from build123d import *

# Parameters (mm, degrees)
SKETCH1_W           = 62.4
SKETCH1_H           = 72.4
SKETCH1_R           = 1.55
SKETCH1_W_2         = 14
BOSS_EXTRUDE1_DEPTH = 1.5
SKETCH3_W           = 14.75
SKETCH3_H           = 25
SKETCH3_W_2         = 12.75
SKETCH3_H_2         = 23
BOSS_EXTRUDE2_DEPTH = 3
SKETCH4_W           = 4
SKETCH4_H           = 4
BOSS_EXTRUDE3_DEPTH = 16.5
SKETCH5_R           = 0.875
CUT_EXTRUDE1_DEPTH  = 4
FILLET1_R           = 1
SKETCH6_R           = 1.55
CUT_EXTRUDE5_DEPTH  = 61.214034909
SKETCH7_W           = 5
SKETCH7_H           = 20
CUT_EXTRUDE3_DEPTH  = 61.214034909
SKETCH8_R           = 1.5
CUT_EXTRUDE4_DEPTH  = 61.64222951
SKETCH9_R           = 1.636711996
CUT_EXTRUDE6_DEPTH  = 61.214034909


with BuildPart() as part:
    # Sketch1 → Boss-Extrude1 (new body)
    # profile 1 of 2: a face of its own
    with BuildSketch(Plane(origin=(0, 0, 0), x_dir=(1, 0, 0), z_dir=(0, 1, 0))):
        Rectangle(SKETCH1_W, SKETCH1_H)
        with Locations(Location((-27.333, -32.333, 0), (0, 0, 270))):
            Circle(SKETCH1_R, mode=Mode.SUBTRACT)
        with Locations(Location((27.333, -32.333, 0), (0, 0, 270))):
            Circle(SKETCH1_R, mode=Mode.SUBTRACT)
        with Locations(Location((-27.333, 32.333, 0), (0, 0, 270))):
            Circle(SKETCH1_R, mode=Mode.SUBTRACT)
        with Locations(Location((27.333, 32.333, 0), (0, 0, 270))):
            Circle(SKETCH1_R, mode=Mode.SUBTRACT)
    # profile 2 of 2: a face of its own
    with BuildSketch(Plane(origin=(0, 0, 0), x_dir=(1, 0, 0), z_dir=(0, 1, 0))):
        with Locations((38.2, 0)):
            Rectangle(SKETCH1_W_2, SKETCH1_H)
    extrude(amount=BOSS_EXTRUDE1_DEPTH)

    # Sketch3 → Boss-Extrude2 (add)
    with BuildSketch(Plane(origin=(0, 1.5, 0), x_dir=(1, 0, 0), z_dir=(0, 1, 0))):
        with Locations((37.825, 0)):
            Rectangle(SKETCH3_W, SKETCH3_H)
        with Locations((37.825, 0)):
            Rectangle(SKETCH3_W_2, SKETCH3_H_2, mode=Mode.SUBTRACT)
    extrude(amount=BOSS_EXTRUDE2_DEPTH)

    # Sketch4 → Boss-Extrude3 (add)
    with BuildSketch(Plane(origin=(0, 1.5, 0), x_dir=(1, 0, 0), z_dir=(0, 1, 0))):
        with Locations((37.825, -14)):
            Rectangle(SKETCH4_W, SKETCH4_H)
        with Locations((37.825, 14.5)):
            Rectangle(SKETCH4_W, SKETCH4_H)
    extrude(amount=BOSS_EXTRUDE3_DEPTH)

    # Sketch5 → Cut-Extrude1 (cut)
    with BuildSketch(Plane(origin=(0, 18, 0), x_dir=(1, 0, 0), z_dir=(0, 1, 0))):
        with Locations(Location((37.825, -14, 0), (0, 0, 270))):
            Circle(SKETCH5_R)
        with Locations(Location((37.825, 14.5, 0), (0, 0, 270))):
            Circle(SKETCH5_R)
    extrude(amount=-CUT_EXTRUDE1_DEPTH, mode=Mode.SUBTRACT)

    # Fillet1
    fillet1_edges = [part.edges().sort_by_distance(p)[0] for p in [
        (42.5125, 1.5, -12.5),
        (30.45, 1.5, 0),
        (33.1375, 1.5, 12.5),
        (42.5125, 1.5, 12.5),
        (35.825, 1.5, 14.25),
        (39.825, 1.5, 14.25),
        (37.825, 1.5, 16),
        (33.1375, 1.5, -12.5),
        (35.825, 1.5, -14.5),
        (39.825, 1.5, -14.5),
        (37.825, 1.5, -16.5),
    ]]
    fillet(fillet1_edges, radius=FILLET1_R)

    # Sketch6 → Cut-Extrude5 (cut, through all)
    with BuildSketch(Plane(origin=(0, 1.5, 0), x_dir=(1, 0, 0), z_dir=(0, 1, 0))):
        with Locations(Location((7.473, -32.333, 0), (0, 0, 270))):
            Circle(SKETCH6_R)
        with Locations(Location((7.473, 32.333, 0), (0, 0, 270))):
            Circle(SKETCH6_R)
    extrude(amount=-CUT_EXTRUDE5_DEPTH, mode=Mode.SUBTRACT)

    # Sketch7 → Cut-Extrude3 (cut, through all)
    with BuildSketch(Plane(origin=(0, 1.5, 0), x_dir=(1, 0, 0), z_dir=(0, 1, 0))):
        with Locations((20, 0)):
            Rectangle(SKETCH7_W, SKETCH7_H)
    extrude(amount=-CUT_EXTRUDE3_DEPTH, mode=Mode.SUBTRACT)

    # Sketch8 → Cut-Extrude4 (cut, through all)
    with BuildSketch(Plane.XZ):
        with Locations(Location((-22.2, -6.73, 0), (0, 0, 270))):
            Circle(SKETCH8_R)
        with Locations(Location((-22.2, 6.73, 0), (0, 0, 270))):
            Circle(SKETCH8_R)
    extrude(amount=-CUT_EXTRUDE4_DEPTH, mode=Mode.SUBTRACT)

    # Sketch9 → Cut-Extrude6 (cut, through all)
    with BuildSketch(Plane(origin=(0, 1.5, 0), x_dir=(1, 0, 0), z_dir=(0, 1, 0))):
        with Locations(Location((-22.2, 6.73, 0), (0, 0, 270))):
            Circle(SKETCH9_R)
        with BuildLine():
            Line((-20.2, 24.2), (-20.2, 18.2))
            ThreePointArc((-20.2, 18.2), (-22.2, 16.2), (-24.2, 18.2))
            Line((-24.2, 18.2), (-24.2, 24.2))
            ThreePointArc((-24.2, 24.2), (-22.2, 26.2), (-20.2, 24.2))
        make_face()
        with BuildLine():
            Line((-20.2, -18.2), (-20.2, -24.2))
            ThreePointArc((-20.2, -24.2), (-22.2, -26.2), (-24.2, -24.2))
            Line((-24.2, -24.2), (-24.2, -18.2))
            ThreePointArc((-24.2, -18.2), (-22.2, -16.2), (-20.2, -18.2))
        make_face()
        with BuildLine():
            Line((10.8, 24.2), (10.8, 18.2))
            ThreePointArc((10.8, 18.2), (12.8, 16.2), (14.8, 18.2))
            Line((14.8, 18.2), (14.8, 24.2))
            ThreePointArc((14.8, 24.2), (12.8, 26.2), (10.8, 24.2))
        make_face()
        with BuildLine():
            Line((10.8, -18.2), (10.8, -24.2))
            ThreePointArc((10.8, -24.2), (12.8, -26.2), (14.8, -24.2))
            Line((14.8, -24.2), (14.8, -18.2))
            ThreePointArc((14.8, -18.2), (12.8, -16.2), (10.8, -18.2))
        make_face()
    extrude(amount=-CUT_EXTRUDE6_DEPTH, mode=Mode.SUBTRACT)


solid = part.part
Geometry check sheet. Reference: the model listing, model coordinates, mm. A direction names the side the tool comes from. Give positions to 0.01 mm unless a question says otherwise; leave off trailing zeros. Loops run counter-clockwise (first coordinate to the right, second up) from the corner with the lowest first, then second, coordinate; pieces in that order, holes last. Notation, with made-up numbers: M 10.5,36.5 L 57.5,36.5 A23 cw 57.5,54.5 Z; hole C 1,13.5 d3. An arc over 180 degrees is marked long. Answer as a JSON object with one key per item and string values. Group by question number.
Item 1: Sectioned sample at A-A on y = 12.25. Record the boundary of the cut face in (x, z) (3 decimals), plus the area to 3 significant figures.
Item 2: Gauge pin test, flat ends, axial feed: pin 1 (2 mm diameter, centred on x = -15.5, z = 0, fed in from +Y); pin 2 (3 mm diameter, centred on x = -22.2, z = -6.73, fed in from -Y); pin 3 (1.6 mm diameter, centred on x = 43.5, y = 3, fed in from +Z); pin 4 (1.1 mm diameter, centred on x = 37.825, z = 14, fed in from -Y). Record the tip position at first contact, or that the pin passes through.
Item 3: Sectioned sample at B-B on z = -6.73. Record the boundary of the cut face in (x, y), plus the area to 3 significant figures.
Item 4: Access from +Z, -Z, +X, -X, +Y, -Y to the whole of each face (thin tool, end or side, straight path). Record for faces 1 (the flat face through (45.2, 2, 1)), 2 (the cylindrical face through (38.693, 16.028, 13.886)), 3 (the flat face through (30.45, 3, 0)), 4 (the flat face through (38, 11, 12)), 5 (the cylindrical face through (12.8, 0.8, -26.2)).
Item 5: Sectioned sample at D-D on z = -14.5. Record the boundary of the cut face in (x, y) (3 decimals), plus the area to 3 significant figures.
Item 6: Sectioned sample at C-C on x = -22.2. Record the boundary of the cut face in (y, z), plus the area to 3 significant figures.
Item 7: Material ranges on L1, parallel to X at y = 0.65, z = -6.73; L2, parallel to Y at x = 33, z = 23; L3, parallel to X at y = 15.5, z = 15 (3 decimals), recorded low to high.
Item 8: Mould release check, pull along Z, two halves, no side actions. Record for faces 6 (the cylindrical face through (-22.2, 0.8, -26.2)), 7 (the flat face through (33, 3, 12.5)), 8 (the flat face through (6, 1.5, -1)), 9 (the flat face through (38, 10, -16.5)): pulls with the +Z half, pulls with the -Z half, needs draft (parallel to the pull), parting line crosses it, or undercut.
Findings below:
{
 "1": {"outline": "M 35.825,-16.5 L 39.825,-16.5 L 39.825,-12.5 L 35.825,-12.5 Z; M 35.825,12 L 39.825,12 L 39.825,16 L 35.825,16 Z", "area": "32.0 mm2"},
 "2": {"pin 1": "y = 1.5", "pin 2": "through", "pin 3": "z = 12.55", "pin 4": "y = 0"},
 "3": {"outline": "M -31.2,0 L -23.84,0 L -23.84,1.5 L -31.2,1.5 Z; M -20.56,0 L 17.5,0 L 17.5,1.5 L -20.56,1.5 Z; M 22.5,0 L 45.2,0 L 45.2,4.5 L 44.2,4.5 L 44.2,1.5 L 31.45,1.5 L 31.45,4.5 L 30.45,4.5 L 30.45,2.5 A1 cw 29.45,1.5 L 22.5,1.5 Z", "area": "108 mm2"},
 "4": {"face 1": "+Z, -Z, +X, +Y, -Y", "face 2": "+Y", "face 3": "+Z, -Z, -X, +Y", "face 4": "+X, -X, +Y", "face 5": "+Y, -Y"},
 "5": {"outline": "M -31.2,0 L 45.2,0 L 45.2,1.5 L 40.825,1.5 A1 cw 39.825,2.5 L 39.825,18 L 38.7,18 L 38.7,14 L 36.95,14 L 36.95,18 L 35.825,18 L 35.825,2.5 A1 cw 34.825,1.5 L -31.2,1.5 Z", "area": "174 mm2"},
 "6": {"outline": "M 0,-36.2 L 1.5,-36.2 L 1.5,-26.2 L 0,-26.2 Z; M 0,-16.2 L 1.5,-16.2 L 1.5,-8.37 L 0,-8.37 Z; M 0,-5.09 L 1.5,-5.09 L 1.5,5.23 L 0,5.23 Z; M 0,8.23 L 1.5,8.23 L 1.5,16.2 L 0,16.2 Z; M 0,26.2 L 1.5,26.2 L 1.5,36.2 L 0,36.2 Z", "area": "69.2 mm2"},
 "7": {"L1": "-31.2 to -23.84, -20.56 to 17.5, 22.5 to 45.2", "L2": "0 to 1.5", "L3": "35.825 to 39.825"},
 "8": {"face 6": "undercut", "face 7": "pulls with the +Z half", "face 8": "needs draft", "face 9": "pulls with the -Z half"}
}
